Could you check a few things on this model? Use its own coordinates, in mm. Face numbers are marked on the shaded views. A direction names the side the tool comes from. Coordinates: 2 decimals unless noted, no trailing zeros. Loops run counter-clockwise (first coordinate to the right, second up) from the corner with the lowest first, then second, coordinate; pieces in that order, holes last. Notation, with made-up numbers: (-10.5, 28) -> (34.5, 28) arc R13 cw to (34.5, 43) -> close; hole circle Ø5 at (79, -17). An arc over 180 degrees is marked (long way). One line per question, with ' | ' between items. Start each with the question number.
(1) Suppose I cut it at A-A (z = 6.75). Please give me the cut outline in (x, y), plus the area to 3 significant figures.
(2) Suppose I cut it at D-D (z = 4). Please give me the cut outline in (x, y).
(3) Which directions (+Z, -Z, +X, -X, +Y, -Y) give clear straight access to the entire face, cutting with the end or side of a thin tool? Please do the marked faces 1 and 2.
(4) I'm going to push flat-ended pins straight in: pin 1 Ø6 at (x, y) = (41.5, 12) entering from -Z; pin 2 Ø1 at (y, z) = (14, 4.5) entering from +X; pin 3 Ø2 at (x, y) = (44, -15) entering from +Z. Where does each tip first touch, or does it pass through?
(5) If I drill on line 1 along Y through (x, z) = (14, 7.8); line 2 along Y through (x, z) = (44, 8.65); line 3 along X through (y, z) = (4, -4.75), over which ranges is the centre line in solid material (lowest first)?
(6) Suppose I cut it at C-C (x = 44). Please give me the cut outline in (y, z).
(7) Suppose I cut it at B-B (y = 0). Please give me the cut outline in (x, z), plus the area to 3 significant figures.
```python
from build123d import *

# Parameters (mm, degrees)
SKETCH1_W           = 20
SKETCH1_H           = 20
BOSS_EXTRUDE1_DEPTH = 4
SKETCH2_R           = 1.1
CUT_EXTRUDE1_DEPTH  = 5
SKETCH3_W           = 4
SKETCH3_H           = 40
BOSS_EXTRUDE2_DEPTH = 45
SKETCH4_R           = 1.25
CUT_EXTRUDE2_DEPTH  = 10
SKETCH5_W           = 4
SKETCH5_H           = 10
BOSS_EXTRUDE4_DEPTH = 4
SKETCH6_W           = 16
SKETCH6_H           = 10
BOSS_EXTRUDE5_DEPTH = 4
CUT_EXTRUDE3_DEPTH  = 4
FILLET6_R           = 8


with BuildPart() as part:
    # Sketch1 → Boss-Extrude1 (new body)
    with BuildSketch(Plane(origin=(0, 0, 0), x_dir=(0, 0, -1), z_dir=(1, 0, 0))):
        Rectangle(SKETCH1_W, SKETCH1_H)
    extrude(amount=BOSS_EXTRUDE1_DEPTH)

    # Sketch2 → Cut-Extrude1 (cut, through all)
    with BuildSketch(Plane(origin=(4, 0, 0), x_dir=(0, 0, -1), z_dir=(1, 0, 0))):
        with Locations((-4.5, 0)):
            Circle(SKETCH2_R)
        with Locations((4.5, 0)):
            Circle(SKETCH2_R)
        with Locations((0, 4.5)):
            Circle(SKETCH2_R)
        with Locations((0, -4.5)):
            Circle(SKETCH2_R)
    extrude(amount=-CUT_EXTRUDE1_DEPTH, mode=Mode.SUBTRACT)

    # Sketch3 → Boss-Extrude2 (add)
    with BuildSketch(Plane(origin=(4, 0, 0), x_dir=(0, 0, -1), z_dir=(1, 0, 0))):
        with Locations((-8, 0)):
            Rectangle(SKETCH3_W, SKETCH3_H)
    extrude(amount=BOSS_EXTRUDE2_DEPTH)

    # Sketch4 → Cut-Extrude2 (cut)
    with BuildSketch(Plane.XY.offset(10)):
        with Locations((14, 15)):
            Circle(SKETCH4_R)
        with Locations((14, -15)):
            Circle(SKETCH4_R)
        with Locations((44, 15)):
            Circle(SKETCH4_R)
        with Locations((44, -15)):
            Circle(SKETCH4_R)
    extrude(amount=-CUT_EXTRUDE2_DEPTH, mode=Mode.SUBTRACT)

    # Sketch5 → Boss-Extrude4 (add)
    with BuildSketch(Plane.ZY.offset(-4)):
        with Locations((8, -15)):
            Rectangle(SKETCH5_W, SKETCH5_H)
        with Locations((8, 15)):
            Rectangle(SKETCH5_W, SKETCH5_H)
    extrude(amount=BOSS_EXTRUDE4_DEPTH)

    # Sketch6 → Boss-Extrude5 (add)
    with BuildSketch(Plane.ZY):
        with Locations((-2, 15)):
            Rectangle(SKETCH6_W, SKETCH6_H)
        with Locations((-2, -15)):
            Rectangle(SKETCH6_W, SKETCH6_H)
    extrude(amount=-BOSS_EXTRUDE5_DEPTH)

    # Sketch7 → Cut-Extrude3 (cut)
    with BuildSketch(Plane.ZY):
        with BuildLine():
            Line((-10, -20), (6, -20))
            ThreePointArc((6, -20), (-7.996256634, 0), (6, 20))
            Line((6, 20), (-10, 20))
            Line((-10, 20), (-10, -20))
        make_face()
    extrude(amount=-CUT_EXTRUDE3_DEPTH, mode=Mode.SUBTRACT)

    # Fillet6
    fillet6_edges = [part.edges().sort_by_distance(p)[0] for p in [
        (49, -20, 8),
        (49, 20, 8),
    ]]
    fillet(fillet6_edges, radius=FILLET6_R)


solid = part.part
```
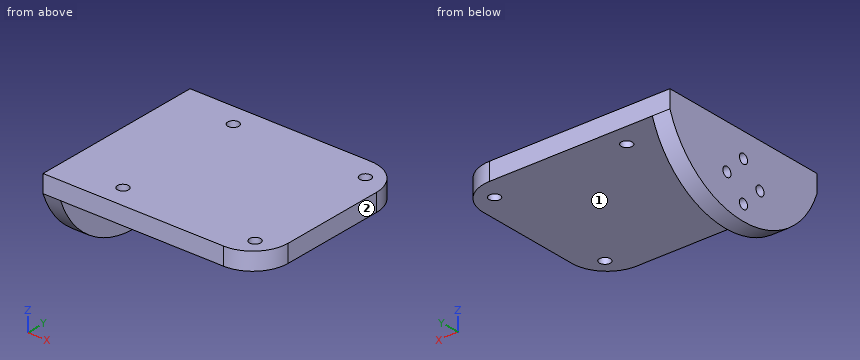
Checks:
1) outline: (0, -20) -> (41, -20) arc R8 ccw to (49, -12) -> (49, 12) arc R8 ccw to (41, 20) -> (0, 20) -> close; hole circle Ø2.5 at (14, -15); hole circle Ø2.5 at (14, 15); hole circle Ø2.5 at (44, -15); hole circle Ø2.5 at (44, 15) | area: 1,910 mm^2
2) outline: (0, -19.15) -> (4, -19.15) -> (4, -0.98) -> (0, -0.98) -> close; (0, 0.98) -> (4, 0.98) -> (4, 19.15) -> (0, 19.15) -> close
3) face 1: -Z, +X, +Y, -Y | face 2: +Z, -Z, +X, +Y, -Y
4) pin 1: stops at z = 6 | pin 2: stops at x = 4 | pin 3: passes through
5) line 1: y = -20 to -16.25, -13.75 to 13.75, 16.25 to 20 | line 2: y = -19.42 to -16.25, -13.75 to 13.75, 16.25 to 19.42 | line 3: x = 0 to 4
6) outline: (-19.42, 6) -> (-16.25, 6) -> (-16.25, 10) -> (-19.42, 10) -> close; (-13.75, 6) -> (13.75, 6) -> (13.75, 10) -> (-13.75, 10) -> close; (16.25, 6) -> (19.42, 6) -> (19.42, 10) -> (16.25, 10) -> close
7) outline: (0, -8) -> (4, -8) -> (4, -5.6) -> (0, -5.6) -> close; (0, -3.4) -> (4, -3.4) -> (4, 3.4) -> (0, 3.4) -> close; (0, 5.6) -> (4, 5.6) -> (4, 6) -> (49, 6) -> (49, 10) -> (0, 10) -> close | area: 234 mm^2
